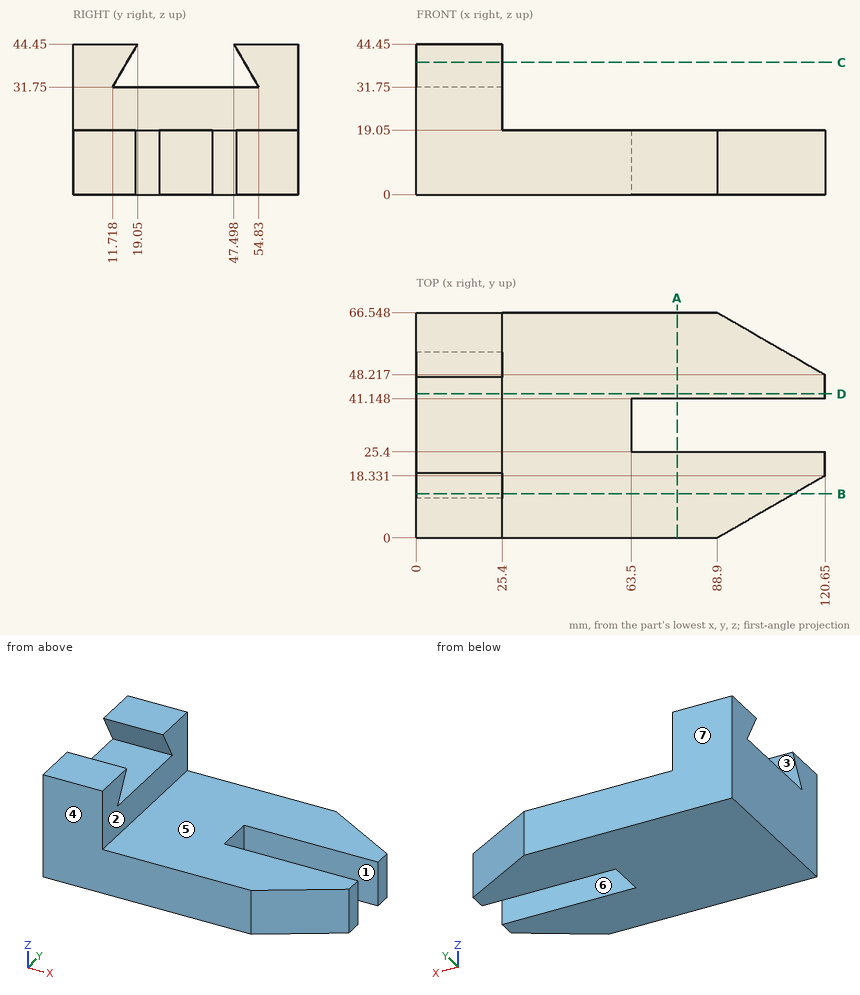
Answer from the drawing. Dimensions are ordinates in mm from the lowest x, y and z of the part. A direction names the side the tool comes from. Coordinates: 2 decimals unless noted, no trailing zeros. Order: outer loops, then holes, each group sorted by start corner. A loop starts at its lowest first (then second) coordinate and runs counter-clockwise, first axis right, second up. Notation, with made-up numbers: (-5.75, -9.5) - (37.25, -9.5) arc R27 cw to (37.25, 26.5) - close; hole circle Ø2 at (49.25, 76). An arc over 180 degrees is marked (long way). Answer as a JSON object with one key per item and string values. Group by question number.
Item 1: Consider probe 1 along Y at (x, z) = (68.5, 7); probe 2 along Z at (x, y) = (93, 22); probe 3 along X at (y, z) = (6.5, 29). Determine where each line is inside the solid, lowest interval first. Write a range as from..to.
Item 2: Section D-D (y = 42.5) is taken. Give the vertices of the cut face in (x, z), plus the area to 3 significant figures.
Item 3: The mould has two halves that part along Y. Classify the marked faces 4, 5, 6 and 7: +Y half, -Y half, draft (parallel to the pull), parting line (faces both ways), or undercut.
Item 4: A tool of negligible diameter and unlimited length cuts with its end or side. For the marked faces 1, 2 and 3, from which of +Z, -Z, +X, -X, +Y, -Y can it reach the whole face along a straight path? Write none if from no direction.
Item 5: Section B-B (y = 13) is taken. Give the vertices of the cut face in (x, z), plus the area to 3 significant figures.
Item 6: Flat-ended cylindrical pins translate along their axes: P1, Ø12, axis at y = 19, z = 32, coming from the +X side; P2, Ø4.5, axis at y = 30.5, z = 10, coming from the +X side; P3, Ø7.5, axis at x = 13, y = 30, coming from the +Z side. Find the tip coordinate at first contact, or state that the pin passes through.
Item 7: Section C-C (z = 39) is taken. Give the vertices of the cut face in (x, y) (1 decimal).
Item 8: Section A-A (x = 77) is taken. Give the vertices of the cut face in (y, z), plus the area to 3 significant figures.
Results are:
{
 "1": {"probe 1": "y = 0..25.4, 41.15..66.55", "probe 2": "z = 0..19.05", "probe 3": "x = 0..25.4"},
 "2": {"outline": "(0, 0) - (120.65, 0) - (120.65, 19.05) - (25.4, 19.05) - (25.4, 31.75) - (0, 31.75) - close", "area": "2,620 mm^2"},
 "3": {"face 4": "-Y half", "face 5": "draft", "face 6": "undercut", "face 7": "+Y half"},
 "4": {"face 1": "+Z, -Z, +X", "face 2": "+Z, +X, +Y, -Y", "face 3": "+X, -X"},
 "5": {"outline": "(0, 0) - (111.42, 0) - (111.42, 19.05) - (25.4, 19.05) - (25.4, 31.75) - (0, 31.75) - close; (0, 33.97) - (25.4, 33.97) - (25.4, 44.45) - (0, 44.45) - close", "area": "2,710 mm^2"},
 "6": {"P1": "stops at x = 25.4", "P2": "stops at x = 63.5", "P3": "stops at z = 31.75"},
 "7": {"outline": "(0, 0) - (25.4, 0) - (25.4, 15.9) - (0, 15.9) - close; (0, 50.6) - (25.4, 50.6) - (25.4, 66.5) - (0, 66.5) - close"},
 "8": {"outline": "(0, 0) - (25.4, 0) - (25.4, 19.05) - (0, 19.05) - close; (41.15, 0) - (66.55, 0) - (66.55, 19.05) - (41.15, 19.05) - close", "area": "968 mm^2"}
}
